Check sheet for the modelled part. Datum: model origin and axes. Units: mm. A direction names the side the tool comes from. Round coordinates to 2 decimals unless told otherwise and drop trailing zeros. Order: outer loops, then holes, each group sorted by start corner. A loop starts at its lowest first (then second) coordinate and runs counter-clockwise, first axis right, second up. Notation, with made-up numbers: (32, 37.5) -> (65, 37.5) arc R11 cw to (65, 47.5) -> close; hole circle Ø9 at (65, -37.5). An arc over 180 degrees is marked (long way). Answer in a Markdown table with one row per item. Add a question column.
1. Depth check by flat-ended pin: P1, Ø1.5, axis at y = 30.5, z = 13.5, coming from the +X side; P2, Ø4, axis at y = 8, z = -5.5, coming from the +X side; P3, Ø6.5, axis at x = 16, z = 1.5, coming from the +Y side. Enter the tip coordinate at first touch or a pass-through.
2. Material ranges on L1, parallel to Z at x = 11, y = 9.5; L2, parallel to X at y = 17, z = -9.5; L3, parallel to X at y = 30.5, z = -13, recorded low to high. Write a range as from..to.
3. Sectioned sample at C-C, the plane z = 8. Record the boundary of the cut face in (x, y).
4. Sectioned sample at A-A, the plane x = 19. Record the boundary of the cut face in (y, z).
5. Sectioned sample at B-B, the plane y = 9. Record the boundary of the cut face in (x, z), then the cut area to 3 significant figures.
6. Access from +Z, -Z, +X, -X, +Y, -Y to the whole of each face (thin tool, end or side, straight path). Record for faces 1 (the flat face through (35, 3, 0)), 2 (the flat face through (13, 13, 11)), 3 (the flat face through (6.7, 32, 13)).
7. Draft check along Z on faces 4 (the flat face through (14, 14, -14.06)), 5 (the flat face through (14, 14, 14.06)), 6 (the flat face through (13, 13, -11)), 7 (the flat face through (0, 17, 0)). Enter one of: +Z half, -Z half, draft (parallel to the pull), parting line (faces both ways), or undercut.
```python
from build123d import *

# Parameters (mm, degrees)
SALIENTE_EXTRUIR1_DEPTH = 14.06
CROQUIS4_W              = 30.3
CROQUIS4_H              = 30.3
CORTAR_EXTRUIR1_DEPTH   = 11


with BuildPart() as part:
    # Croquis1 → Saliente-Extruir1 (new body, symmetric)
    with BuildSketch(Plane.XY):
        Polygon((0, 0), (0, 35), (6.7, 35), (6.7, 29), (29, 6.7), (35, 6.7), (35, 0), align=None)
    extrude(amount=SALIENTE_EXTRUIR1_DEPTH, both=True)

    # Croquis4 → Cortar-Extruir1 (cut, symmetric)
    with BuildSketch(Plane.XY):
        with Locations((19.85, 19.85)):
            Rectangle(CROQUIS4_W, CROQUIS4_H)
    extrude(amount=CORTAR_EXTRUIR1_DEPTH, both=True, mode=Mode.SUBTRACT)


solid = part.part
```
Answer key:
| question | item | result |
|---|---|---|
| 1 | P1 | stops at x = 6.7 |
| 1 | P2 | stops at x = 4.7 |
| 1 | P3 | stops at y = 4.7 |
| 2 | L1 | z = -14.06..-11, 11..14.06 |
| 2 | L2 | x = 0..4.7 |
| 2 | L3 | x = 0..6.7 |
| 3 | outline | (0, 0) -> (35, 0) -> (35, 4.7) -> (4.7, 4.7) -> (4.7, 35) -> (0, 35) -> close |
| 4 | outline | (0, -14.06) -> (16.7, -14.06) -> (16.7, -11) -> (4.7, -11) -> (4.7, 11) -> (16.7, 11) -> (16.7, 14.06) -> (0, 14.06) -> close |
| 5 | outline | (0, -14.06) -> (26.7, -14.06) -> (26.7, -11) -> (4.7, -11) -> (4.7, 11) -> (26.7, 11) -> (26.7, 14.06) -> (0, 14.06) -> close |
| 5 | area | 267 mm² |
| 6 | face 1 | +Z, -Z, +X, +Y, -Y |
| 6 | face 2 | +X, +Y |
| 6 | face 3 | +Z, -Z, +X, +Y |
| 7 | face 4 | -Z half |
| 7 | face 5 | +Z half |
| 7 | face 6 | undercut |
| 7 | face 7 | draft |
